Can you work these out from the model? Positions are in its coordinate system, mm. A direction names the side the tool comes from. Coordinates: 2 decimals unless noted, no trailing zeros. Loops run counter-clockwise (first coordinate to the right, second up) from the corner with the lowest first, then second, coordinate; pieces in that order, holes last. Notation, with made-up numbers: M 72,-20.5 L 123,-20.5 A30 cw 123,2.5 Z; hole C 66,87.25 d11. An arc over 180 degrees is marked long. Answer as a JSON object with one key per item and string values. Group by question number.
Item 1: We'd pull the mould along Y, two halves only. Please class faces 3 (the flat face through (-3, 15.24, 3)), 4 (the cylindrical face through (5.014, 7.682, -2.608)), 5 (the cylindrical face through (3.04, 7.73, 0.67)), 6 (the flat face through (-3, 3.175, 5)): +Y half, -Y half, draft (parallel to the pull), parting line (faces both ways), or undercut.
Item 2: I'm going to push flat-ended pins straight in: pin 1 Ø3 at (y, z) = (13.5, 3) entering from +X; pin 2 Ø1 at (y, z) = (3.5, 3.5) entering from -X; pin 3 Ø4 at (x, y) = (-7.5, 1.5) entering from +Z. Where does each tip first touch, or does it pass through?
Item 3: Suppose I cut it at A-A (x = 0). Write out the boundary of the cut face in (y, z) (1 decimal).
Item 4: Suppose I cut it at B-B (z = 0). Write out the boundary of the cut face in (x, y) (1 decimal), then the cut area to 3 significant figures.
Item 5: If I drill on line 1 (Y direction, x = 6.25, z = -1.75) (3 decimals); line 2 (X direction, y = 3.5, z = 0); line 3 (X direction, y = 12.75, z = -8.89), over which ranges is the centre line in solid material (lowest first)?
Item 6: Which directions (+Z, -Z, +X, -X, +Y, -Y) give clear straight access to the entire face, cutting with the end or side of a thin tool? Please do faces 1 (the flat face through (-3, 12.065, 5)), 2 (the cylindrical face through (0.38, 13.67, -7.68)).
Item 7: Suppose I cut it at D-D (x = -8.25). Write out the boundary of the cut face in (y, z) (3 decimals).
Item 8: Suppose I cut it at C-C (z = -9.5). Write out the boundary of the cut face in (x, y) (3 decimals), then the cut area to 3 significant figures.
```python
from build123d import *

# Parameters (mm, degrees)
SKETCH1_R           = 5.6515
SKETCH1_R_2         = 3.1115
BOSS_EXTRUDE1_DEPTH = 7.62
SKETCH1_4_R         = 12.7
SKETCH1_4_R_2       = 5.6515
SKETCH1_4_R_3       = 1.27
BOSS_EXTRUDE2_DEPTH = 3.175


with BuildPart() as part:
    # Sketch1 → Boss-Extrude1 (new body)
    with BuildSketch(Plane(origin=(0, 0, 0), x_dir=(1, 0, 0), z_dir=(0, 1, 0))):
        with Locations(Location((0, 0, 0), (0, 0, 90))):
            Circle(SKETCH1_R)
        with Locations(Location((0, 0, 0), (0, 0, 90))):
            Circle(SKETCH1_R_2, mode=Mode.SUBTRACT)
    boss_extrude1 = extrude(amount=BOSS_EXTRUDE1_DEPTH)

    # Sketch1_4 → Boss-Extrude2 (add)
    with BuildSketch(Plane(origin=(0, 0, 0), x_dir=(1, 0, 0), z_dir=(0, 1, 0))):
        with Locations(Location((0, 0, 0), (0, 0, 270))):
            Circle(SKETCH1_4_R)
        with Locations(Location((0, 0, 0), (0, 0, 90))):
            Circle(SKETCH1_4_R_2, mode=Mode.SUBTRACT)
        with Locations(Location((0, 8.89, 0), (0, 0, 270))):
            Circle(SKETCH1_4_R_3, mode=Mode.SUBTRACT)
    boss_extrude2 = extrude(amount=BOSS_EXTRUDE2_DEPTH)

    # Mirror1: Boss-Extrude1, Boss-Extrude2 across plane
    add(boss_extrude1.mirror(Plane.ZX.offset(7.62)))
    add(boss_extrude2.mirror(Plane.ZX.offset(7.62)))


solid = part.part
```
From the geometry:
{
 "1": {"face 3": "+Y half", "face 4": "undercut", "face 5": "draft", "face 6": "undercut"},
 "2": {"pin 1": "x = 12.61", "pin 2": "x = -12.31", "pin 3": "z = 11.45"},
 "3": {"outline": "M 0,-12.7 L 3.2,-12.7 L 3.2,-10.2 L 0,-10.2 Z; M 0,-7.6 L 3.2,-7.6 L 3.2,-5.7 L 12.1,-5.7 L 12.1,-7.6 L 15.2,-7.6 L 15.2,-3.1 L 0,-3.1 Z; M 0,3.1 L 15.2,3.1 L 15.2,12.7 L 12.1,12.7 L 12.1,5.7 L 3.2,5.7 L 3.2,12.7 L 0,12.7 Z; M 12.1,-12.7 L 15.2,-12.7 L 15.2,-10.2 L 12.1,-10.2 Z"},
 "4": {"outline": "M -12.7,0 L -3.1,0 L -3.1,15.2 L -12.7,15.2 L -12.7,12.1 L -5.7,12.1 L -5.7,3.2 L -12.7,3.2 Z; M 3.1,0 L 12.7,0 L 12.7,3.2 L 5.7,3.2 L 5.7,12.1 L 12.7,12.1 L 12.7,15.2 L 3.1,15.2 Z", "area": "167 mm2"},
 "5": {"line 1": "0 to 3.175, 12.065 to 15.24", "line 2": "-5.65 to -3.11, 3.11 to 5.65", "line 3": "-9.07 to -1.27, 1.27 to 9.07"},
 "6": {"face 1": "none", "face 2": "+Y, -Y"},
 "7": {"outline": "M 0,-9.655 L 3.175,-9.655 L 3.175,9.655 L 0,9.655 Z; M 12.065,-9.655 L 15.24,-9.655 L 15.24,9.655 L 12.065,9.655 Z"},
 "8": {"outline": "M -8.429,0 L -1.114,0 L -1.114,3.175 L -8.429,3.175 Z; M -8.429,12.065 L -1.114,12.065 L -1.114,15.24 L -8.429,15.24 Z; M 1.114,0 L 8.429,0 L 8.429,3.175 L 1.114,3.175 Z; M 1.114,12.065 L 8.429,12.065 L 8.429,15.24 L 1.114,15.24 Z", "area": "92.9 mm2"}
}
